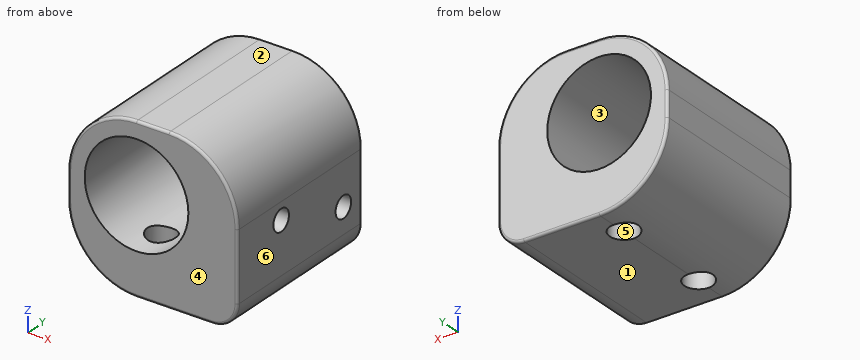
from build123d import *

# Parameters (mm, degrees)
SKETCH_1_R             = 6.05
EXTRUDE_1_DEPTH        = 20
SKETCH_2_R             = 1
CUT_EXTRUDE_1_DEPTH    = 2
HOLE_WIZARD_M3_1_D     = 2.5
HOLE_WIZARD_M3_1_DEPTH = 7
HOLE_WIZARD_M3_1_TIP   = 0.751075774
HOLE_WIZARD_M4_1_D     = 3.3
HOLE_WIZARD_M4_1_DEPTH = 11.5
HOLE_WIZARD_M4_1_TIP   = 0.991420021
FILLET_1_R             = 0.3


with BuildPart() as part:
    # 草图1 → 凸台-拉伸1 (new body)
    with BuildSketch(Plane(origin=(0, 0, 0), x_dir=(1, 0, 0), z_dir=(0, 1, 0))):
        with BuildLine():
            Line((0, 11), (8.8, 11))
            ThreePointArc((8.8, 11), (10.921320344, 10.121320344), (11.8, 8))
            Line((11.8, 8), (11.8, 0))
            ThreePointArc((11.8, 0), (9.456854249, -5.656854249), (3.8, -8))
            Line((3.8, -8), (0, -8))
            ThreePointArc((0, -8), (-5.656854249, -5.656854249), (-8, 0))
            Line((-8, 0), (-8, 3))
            ThreePointArc((-8, 3), (-5.656854249, 8.656854249), (0, 11))
        make_face()
        Circle(SKETCH_1_R, mode=Mode.SUBTRACT)
    extrude(amount=EXTRUDE_1_DEPTH)

    # 草图2 → 切除-拉伸1 (cut)
    with BuildSketch(Plane(origin=(11.8, 0, 0), x_dir=(0, 0, -1), z_dir=(1, 0, 0))):
        with Locations((5, 17)):
            Circle(SKETCH_2_R)
        with Locations((2, 7)):
            Circle(SKETCH_2_R)
    extrude(amount=-CUT_EXTRUDE_1_DEPTH, mode=Mode.SUBTRACT)

    # M3 螺纹孔1
    with Locations(Plane(origin=(11.8, 0, 0), x_dir=(0, 0, -1), z_dir=(1, 0, 0))):
        with Locations((5, 17), (2, 7)):
            Hole(HOLE_WIZARD_M3_1_D / 2, depth=HOLE_WIZARD_M3_1_DEPTH)
            with Locations((0, 0, -(HOLE_WIZARD_M3_1_DEPTH + HOLE_WIZARD_M3_1_TIP / 2))):  # 118° drill point
                Cone(0, HOLE_WIZARD_M3_1_D / 2, HOLE_WIZARD_M3_1_TIP, mode=Mode.SUBTRACT)

    # M4 螺纹孔1
    with Locations(Plane(origin=(3, 0, -11), x_dir=(1, 0, 0), z_dir=(0, 0, -1))):
        with Locations((-3, -16), (-3, -4)):
            Hole(HOLE_WIZARD_M4_1_D / 2, depth=HOLE_WIZARD_M4_1_DEPTH)
            with Locations((0, 0, -(HOLE_WIZARD_M4_1_DEPTH + HOLE_WIZARD_M4_1_TIP / 2))):  # 118° drill point
                Cone(0, HOLE_WIZARD_M4_1_D / 2, HOLE_WIZARD_M4_1_TIP, mode=Mode.SUBTRACT)

    # 圆角1
    fillet_1_edges = [part.edges().sort_by_distance(p)[0] for p in [
        (10.921320344, 20, -10.121320344),
        (11.8, 0, -4),
        (9.456854249, 0, 5.656854249),
        (4.4, 20, -11),
        (-5.656854249, 20, -8.656854249),
        (-8, 20, -1.5),
        (-5.656854249, 20, 5.656854249),
        (1.9, 20, 8),
        (9.456854249, 20, 5.656854249),
        (11.8, 20, -4),
        (1.9, 0, 8),
        (-5.656854249, 0, 5.656854249),
        (-8, 0, -1.5),
        (-5.656854249, 0, -8.656854249),
        (4.4, 0, -11),
        (10.921320344, 0, -10.121320344),
    ]]
    fillet(fillet_1_edges, radius=FILLET_1_R)


solid = part.part
Verification items for the finished model (mm, model axes). Face numbers are marked on the shaded views. A direction names the side the tool comes from. Coordinates: 2 decimals unless noted, no trailing zeros. Order: outer loops, then holes, each group sorted by start corner. A loop starts at its lowest first (then second) coordinate and runs counter-clockwise, first axis right, second up.
1. Sectioned sample at D-D, the plane x = -0.5. Give the number of separate pieces and of enclosed holes in the cut face, and give its area (3 significant figures).
Results found:
separate pieces: 4
enclosed holes: 0
area: 107 mm2
2. Sectioned sample at A-A, the plane y = 10. Record the cut outline in (x, z).
Results found:
outline: (-8, -3) arc R8 ccw to (0, -11) - (8.8, -11) arc R3 ccw to (11.8, -8) - (11.8, 0) arc R8 ccw to (3.8, 8) - (0, 8) arc R8 ccw to (-8, 0) - close; hole circle Ø12.1 at (0, 0)
3. Release check for a two-part mould opening along Z. For the marked faces 1, 2, 3 and 4 record: +Z half, -Z half, draft (parallel to the pull), parting line (faces both ways), or undercut.
Results found:
face 1: -Z half
face 2: +Z half
face 3: undercut
face 4: draft
4. Scan lines: line 1 (Y direction, x = 0, z = -8.8); line 2 (Y direction, x = 8.75, z = -5); line 3 (Y direction, x = 0.75, z = -9). Record each from-to range of solid material in increasing order.
Results found:
line 1: y = 0 to 2.35, 5.65 to 14.35, 17.65 to 20
line 2: y = 0 to 15.75, 18.25 to 20
line 3: y = 0 to 2.53, 5.47 to 14.53, 17.47 to 20
5. Set-up check for the marked faces 5 and 6: record each of +Z, -Z, +X, -X, +Y, -Y from which the full face is reachable in a straight line by a thin tool's end or side.
Results found:
face 5: -Z
face 6: +Z, -Z, +X, +Y, -Y
6. Sectioned sample at B-B, the plane z = -2. Record the cut outline in (x, y), and give its area (3 significant figures).
Results found:
outline: (-8, 0.3) arc R0.3 ccw to (-7.7, 0) - (-5.71, 0) - (-5.71, 20) - (-7.7, 20) arc R0.3 ccw to (-8, 19.7) - close; (5.71, 0) - (11.5, 0) arc R0.3 ccw to (11.8, 0.3) - (11.8, 5.75) - (5.71, 5.75) - close; (5.71, 8.25) - (11.8, 8.25) - (11.8, 19.7) arc R0.3 ccw to (11.5, 20) - (5.71, 20) - close
area: 152 mm2
7. Go/stop test with flat-tipped pins: pin 1 Ø2 at (y, z) = (8, 3) entering from -X; pin 2 Ø3 at (x, y) = (4, 4.5) entering from +Z; pin 3 Ø2 at (x, y) = (0, 4) entering from -Z; pin 4 Ø5 at (y, z) = (16, -6) entering from -X. Record where each tip stops, or that it passes through.
Results found:
pin 1: stops at x = -7.75
pin 2: stops at z = 8
pin 3: stops at z = 5.97
pin 4: stops at x = -7.98
8. Sectioned sample at C-C, the plane y = 7. Record the cut outline in (x, z), and give its area (3 significant figures).
Results found:
outline: (-8, -3) arc R8 ccw to (0, -11) - (8.8, -11) arc R3 ccw to (11.8, -8) - (11.8, -3.25) - (5.1, -3.25) arc R6.05 cw (long way) to (6, -0.75) - (11.8, -0.75) - (11.8, 0) arc R8 ccw to (3.8, 8) - (0, 8) arc R8 ccw to (-8, 0) - close
area: 203 mm2
